For this review, take the finished solid that the model builds, in its own axes (mm). A direction names the side the tool comes from. Give positions to 0.01 mm unless a question says otherwise; leave off trailing zeros. Write each loop counter-clockwise with the first axis right and the second up, starting at its lowest first coordinate (ties: lowest second). Pieces come first, ordered by that corner, then holes.
1) Draft analysis for pull direction Y (two halves, no side actions). For faces 1 (the face through (0, 0, 0)), 2 (the face through (11.207, 3.529, 11.339)), 3 (the face through (0, 0, -4)), state which applies: pulls with the +Y half, pulls with the -Y half, needs draft (parallel to the pull), parting line crosses it, or undercut.
2) Wall thickness on line 1 along Y through (x, z) = (0, 19.5); line 2 along Z through (x, y) = (-8.25, -0.25); line 3 along X through (y, z) = (6, 0.5): over which ranges is each line inside the solid? List them lowest first.
3) Machinability: for faces 4 (the face through (-2.75, -12.4, -0.99)), 5 (the face through (-2.17, -9.76, 12.2)), which of the approach directions +Z, -Z, +X, -X, +Y, -Y give a long, thin tool a straight path to every point of the face, cutting with its end or side? Answer none if there is none.
4) We need section C-C on z = 13. Give the boundary of the cut face in (x, y).
5) We need section A-A on y = 0. Give the boundary of the cut face in (x, z).
6) For P1, Ø3, axis at y = 7.5, z = 0.5, coming from the -X side; P2, Ø3, axis at x = 3, y = -6, coming from the +Z side; P3, Ø8, axis at x = 5.5, z = 5.5, coming from the +Y side, all flat-tipped, find the tip position at first contact; note any pin that passes through.
from build123d import *

# Parameters (mm, degrees)
F0_R     = 12.7
F0_R_2   = 11.75
F0_R_3   = 10
F1_DEPTH = 4
F2_DEPTH = 25


# Not quite as in the source:
# - a fillet or chamfer that OpenCascade refuses, or shapes differently, is made with other operations: its cross-section is extruded or revolved along the edge and cut away or added


with BuildPart() as f1:
    # F0 (on Top) → F1 (new body)
    with BuildSketch(Plane.XY):
        Circle(F0_R)
        Circle(F0_R_2, mode=Mode.SUBTRACT)
        Circle(F0_R_2)
        Circle(F0_R_3, mode=Mode.SUBTRACT)
        Circle(F0_R_3)
    extrude(amount=-F1_DEPTH)

    # F0 (on Top) → F2 (join)
    with BuildSketch(Plane.XY):
        Circle(F0_R_2)
        Circle(F0_R_3, mode=Mode.SUBTRACT)
    extrude(amount=F2_DEPTH)

    # F3: chamfer of 2 on 2 edges, made by hand

    # F3_s1 → F3_t2 (revolve, cut)
    with BuildSketch(Plane.XZ):
        Polygon((11.75, 23), (9.75, 25), (11.75, 25), align=None)
    revolve(axis=Axis((0, 0, 25), (0, 0, 1)), mode=Mode.SUBTRACT)

    # F3_s3 → F3_t4 (revolve, cut)
    with BuildSketch(Plane.XZ):
        Polygon((12.7, -2), (10.7, -4), (12.7, -4), align=None)
    revolve(axis=Axis((0, 0, -4), (0, 0, 1)), mode=Mode.SUBTRACT)


solid = f1.part
Results list:
1. face 1: undercut
1. face 2: parting line crosses it
1. face 3: needs draft
2. line 1: y = -11.75 to -10, 10 to 11.75
2. line 2: z = -4 to 0
2. line 3: x = -10.1 to -8, 8 to 10.1
3. face 4: +Z, -Z
3. face 5: +Z
4. outline: circle Ø23.5 at (0, 0); hole circle Ø20 at (0, 0)
5. outline: (-12.7, -2) - (-10.7, -4) - (10.7, -4) - (12.7, -2) - (12.7, 0) - (11.75, 0) - (11.75, 23) - (10, 24.75) - (10, 0) - (-10, 0) - (-10, 24.75) - (-11.75, 23) - (-11.75, 0) - (-12.7, 0) - close
6. P1: stops at x = -11.15
6. P2: stops at z = 0
6. P3: stops at y = 11.65
